Source: CAD feature listing. Evaluate the final solid. Frame: model axes, mm. A direction names the side the tool comes from. Round coordinates to 2 decimals unless told otherwise and drop trailing zeros. Order: outer loops, then holes, each group sorted by start corner. A loop starts at its lowest first (then second) coordinate and runs counter-clockwise, first axis right, second up. Notation, with made-up numbers: (23, 20) -> (29, 20) arc R18 ccw to (29, 46) -> close; hole circle Ø8 at (50, -38). An arc over 180 degrees is marked (long way). Answer as CSV lines item,"result".
from build123d import *

# Parameters (mm, degrees)
SKETCH_W     = 25
SKETCH_H     = 25
SKETCH_R     = 7.56
PAD_DEPTH    = 3
SKETCH001_R  = 5.03
PAD001_DEPTH = 9


with BuildPart() as part:
    # Sketch → Pad (new body)
    with BuildSketch(Plane.XY):
        Rectangle(SKETCH_W, SKETCH_H)
        with Locations((-3.608525, 3.489298)):
            Circle(SKETCH_R, mode=Mode.SUBTRACT)
    extrude(amount=PAD_DEPTH)

    # Sketch001 → Pad001 (join)
    with BuildSketch(Plane.XY):
        with Locations((7.418324, -7.412742)):
            Circle(SKETCH001_R)
    extrude(amount=PAD001_DEPTH)


solid = part.part
1. Line query: L1, parallel to Z at x = -3, y = -9; L2, parallel to Y at x = -6, z = 2; L3, parallel to X at y = 2.5, z = 0.5. Output: solid intervals per line, ascending. Write a range as [from, to].
Results below:
L1,"[0, 3]"
L2,"[-12.5, -3.68], [10.66, 12.5]"
L3,"[-12.5, -11.1], [3.89, 12.5]"
2. Section query B-B on y = -3.75. Return loops of the section in (x, z), and give its area (3 significant figures).
Results below:
outline,"(-12.5, 0) -> (-5.79, 0) -> (-5.79, 3) -> (-12.5, 3) -> close; (-1.43, 0) -> (12.5, 0) -> (12.5, 3) -> (10.87, 3) -> (10.87, 9) -> (3.97, 9) -> (3.97, 3) -> (-1.43, 3) -> close"
area,"103 mm2"
3. Section query D-D on x = -4. Return loops of the section in (y, z).
Results below:
outline,"(-12.5, 0) -> (-4.06, 0) -> (-4.06, 3) -> (-12.5, 3) -> close; (11.04, 0) -> (12.5, 0) -> (12.5, 3) -> (11.04, 3) -> close"
4. Section query C-C on y = -7. Return loops of the section in (x, z), and give its area (3 significant figures).
Results below:
outline,"(-12.5, 0) -> (12.5, 0) -> (12.5, 3) -> (12.43, 3) -> (12.43, 9) -> (2.41, 9) -> (2.41, 3) -> (-12.5, 3) -> close"
area,"135 mm2"
5. Pin query (flat end, axial travel): pin 1 (4 mm diameter, centred on x = 5, z = 7.5, fed in from -Y); pin 2 (1 mm diameter, centred on y = -6.5, z = 7.5, fed in from +X); pin 3 (3 mm diameter, centred on x = 3, y = -1.5, fed in from +Z). Return the tip coordinate at first contact, or that it passes through.
Results below:
pin 1,"y = -12.43"
pin 2,"x = 12.43"
pin 3,"z = 3"
6. Mould query, pull axis Y, two halves, no side actions, for faces 3 (the flat face through (3, -3, 3)), 4 (the flat face through (0, -12.5, 1)), 5 (the cylindrical face through (3.602, 5.76, 1.479)). Classes: released by +Y, released by -Y, zero draft, split by the parting line, or undercut.
Results below:
face 3,"zero draft"
face 4,"released by -Y"
face 5,"undercut"
7. Reachability of faces 1 (the cylindrical face through (12.216, -5.902, 5.958)), 2 (the flat face through (7, -7, 9)) from +Z, -Z, +X, -X, +Y, -Y: full face, straight path, thin tool, end or side. Return the list, or none.
Results below:
face 1,"+Z"
face 2,"+Z, +X, -X, +Y, -Y"
8. Section query A-A on x = 1.5. Return loops of the section in (y, z).
Results below:
outline,"(-12.5, 0) -> (-2.08, 0) -> (-2.08, 3) -> (-12.5, 3) -> close; (9.06, 0) -> (12.5, 0) -> (12.5, 3) -> (9.06, 3) -> close"
